from build123d import *

# Parameters (mm, degrees)
F0_W      = 38.1
F0_H      = 38.1
F1_DEPTH  = 38.1
F6_DEPTH  = 38.1
F7_W      = 4.854846
F7_H      = 38.1
F8_DEPTH  = 38.1
F9_W      = 19.943573
F9_H      = 10.434402
F9_W_2    = 13.076427
F9_W_3    = 38.1
F9_H_2    = 6.627924
F9_H_3    = 10.877674
F10_DEPTH = 38.1


with BuildPart() as f1:
    # F0 (on Front) → F1 (new body)
    with BuildSketch(Plane.XZ):
        with Locations((19.05, 19.05)):
            Rectangle(F0_W, F0_H)
    extrude(amount=F1_DEPTH)

    # F5 (on offset) → F6 (cut)
    with BuildSketch(Plane.XZ.offset(38.1)):
        Polygon((0, 38.1), (0, 0), (6.35, 38.1), align=None)
        Polygon((25.4, 38.1), (12.7, 38.1), (19.05, 22.225), align=None)
        Polygon((31.75, 38.1), (38.1, 0), (38.1, 38.1), align=None)
        Polygon((11.43, 22.225), (6.35, 0), (31.75, 0), (26.67, 22.225), (21.59, 9.525), (16.51, 9.525), align=None)
    extrude(amount=-F6_DEPTH, mode=Mode.SUBTRACT)

    # F7 (on offset) → F8 (cut)
    with BuildSketch(Plane.YZ.offset(38.1)):
        with Locations((-35.672577, 19.05)):
            Rectangle(F7_W, F7_H)
        Polygon((-19.05, 0), (0, 0), (0, 38.1), (-19.05, 38.1), (-13.519695, 34.353327), (-10.860084, 29.699003), (-10.860084, 19.725459), (-10.860084, 13.076427), (-10.860084, 6.427397), (-13.962964, 2.216344), align=None)
    extrude(amount=-F8_DEPTH, mode=Mode.SUBTRACT)

    # F9 (on offset) → F10 (cut)
    with BuildSketch(Plane.XY.offset(38.1)):
        with Locations((28.128214, -21.174875)):
            Rectangle(F9_W, F9_H)
        with Locations((6.538213, -21.174875)):
            Rectangle(F9_W_2, F9_H)
        with Locations((19.05, -34.786038)):
            Rectangle(F9_W_3, F9_H_2)
        with Locations((19.05, -5.438837)):
            Rectangle(F9_W_3, F9_H_3)
    extrude(amount=-F10_DEPTH, mode=Mode.SUBTRACT)


solid = f1.part
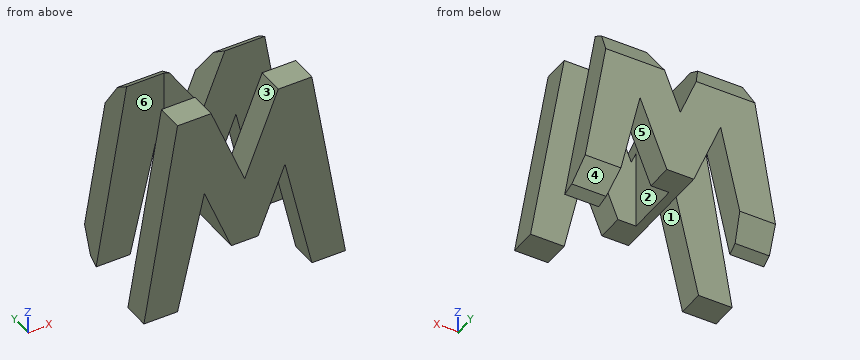
The model under review builds one solid part; all positions refer to its coordinate system, in mm. Face numbers are marked on the shaded views. A direction names the side the tool comes from. Give positions to 0.01 mm unless a question says otherwise; leave off trailing zeros. Write each loop counter-clockwise with the first axis right and the second up, starting at its lowest first coordinate (ties: lowest second). Pieces come first, ordered by that corner, then holes. Notation, with made-up numbers: M 8,-33.75 L 42,-33.75 A23 ccw 42,2.25 Z; hole C 53,11 d11. An arc over 180 degrees is marked long. One line per question, with ' | ' between items. Start each with the question number.
Item 1: For pin 1 (12 mm diameter, centred on x = 32.5, y = -13, fed in from -Z); pin 2 (2 mm diameter, centred on y = -22, z = 27.5, fed in from -X); pin 3 (8 mm diameter, centred on x = 28.5, z = 9, fed in from -Y); pin 4 (3 mm diameter, centred on y = -29.5, z = 19.5, fed in from +X), all flat-tipped, find the tip position at first contact; note any pin that passes through.
Item 2: For the marked faces 1, 2 and 3, list the 3-axis set-ups (+Z, -Z, +X, -X, +Y, -Y) from which the entire face can be reached by the end or side of a thin tool; tool diameter is ignored.
Item 3: We need section D-D on y = -29.5. Write out the cut boundary in (x, z) (3 decimals), plus the area to 3 significant figures.
Item 4: Wall thickness on line 1 (Y direction, x = 22, z = 15.5); line 2 (X direction, y = -27, z = 26); line 3 (X direction, y = -19.5, z = 20): over which ranges is each line inside the solid? List them lowest first. Write a range as from..to.
Item 5: Draft analysis for pull direction Y (two halves, no side actions). For the marked faces 4, 5 and 6, state which applies: released by +Y, released by -Y, zero draft, split by the parting line, or undercut.
Item 6: We need section A-A on x = 26. Write out the cut boundary in (y, z) (3 decimals).
Item 7: We need section C-C on z = 4. Write out the cut boundary in (x, y), plus the area to 3 significant figures.
Item 8: We need section B-B on z = 14.5. Write out the cut boundary in (x, y).
Results found:
1) pin 1: stops at z = 1.35 | pin 2: stops at x = 13.08 | pin 3: stops at y = -31.47 | pin 4: stops at x = 35.1
2) face 1: -Z, +Y, -Y | face 2: +Z, -Z, +X | face 3: +Z, +Y, -Y
3) outline: M 0,0 L 6.35,0 L 11.43,22.225 L 16.51,9.525 L 21.59,9.525 L 26.67,22.225 L 31.75,0 L 38.1,0 L 31.75,38.1 L 25.4,38.1 L 19.05,22.225 L 12.7,38.1 L 6.35,38.1 Z | area: 786 mm2
4) line 1: y = -31.47..-26.39, -15.96..-10.88 | line 2: x = 4.33..17.54, 20.56..33.77 | line 3: x = 13.08..18.16
5) face 4: released by +Y | face 5: zero draft | face 6: undercut
6) outline: M -31.472,20.55 L -26.392,20.55 L -26.392,38.1 L -31.472,38.1 Z; M -15.958,20.55 L -10.878,20.55 L -10.878,29.73 L -13.52,34.353 L -15.958,36.005 Z
7) outline: M 0.67,-31.47 L 7.26,-31.47 L 7.26,-26.39 L 0.67,-26.39 Z; M 0.67,-15.96 L 7.26,-15.96 L 7.26,-12.65 L 0.67,-12.65 Z; M 30.84,-31.47 L 37.43,-31.47 L 37.43,-26.39 L 30.84,-26.39 Z; M 30.84,-15.96 L 37.43,-15.96 L 37.43,-12.65 L 30.84,-12.65 Z | area: 111 mm2
8) outline: M 2.42,-31.47 L 9.66,-31.47 L 9.66,-26.39 L 2.42,-26.39 Z; M 2.42,-15.96 L 9.66,-15.96 L 9.66,-10.88 L 2.42,-10.88 Z; M 14.52,-31.47 L 23.58,-31.47 L 23.58,-26.39 L 18.16,-26.39 L 18.16,-15.96 L 23.58,-15.96 L 23.58,-10.88 L 14.52,-10.88 Z; M 28.44,-31.47 L 35.68,-31.47 L 35.68,-26.39 L 28.44,-26.39 Z; M 28.44,-15.96 L 35.68,-15.96 L 35.68,-10.88 L 28.44,-10.88 Z
